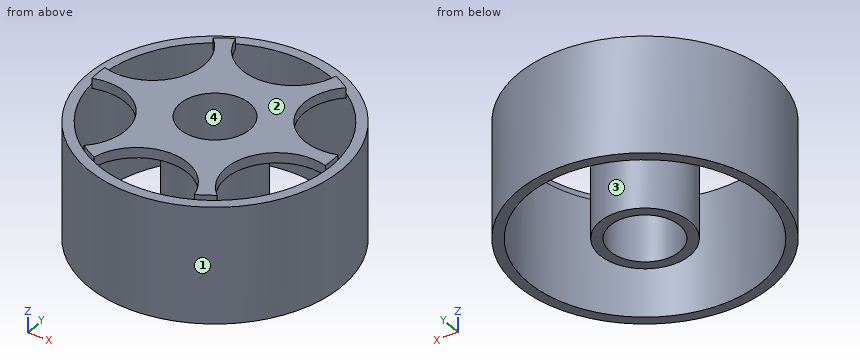
Autodesk Inventor part; units mm, degrees
ref_plane "YZ Plane" through (0, 0, 0) normal (1, 0, 0) x (0, 1, 0)
ref_plane "XZ Plane" through (0, 0, 0) normal (0, 1, 0) x (-1, 0, 0)
ref_plane "XY Plane" through (0, 0, 0) normal (0, 0, 1) x (1, 0, 0)
sketch "Sketch1" plane through (0, 0, 0) normal (0, 0, 1) x (1, 0, 0)
  circle A0 centre (0, 0) radius 5.588
  circle A1 centre (0, 0) radius 4.318
  circle A2 centre (0, 0) radius 14.478
  circle A3 centre (0, 0) radius 15.748
  dimension "d0" = 11.176
  dimension "d1" = 1.27
  dimension "d2" = 8.89
  dimension "d3" = 1.27
extrude "Extrusion1" add sketch "Sketch1" along normal blind 14.478
ref_plane "Work Plane1" through (0, 0, 14.478) normal (0, 0, 1) x (1, 0, 0)
sketch "Sketch2" plane through (0, 0, 14.478) normal (0, 0, 1) x (1, 0, 0)
  circle A0 centre (0, 0) radius 14.478
  circle A1 centre (0, 0) radius 15.748
  circle A2 centre (0, 0) radius 4.318
  circle A3 centre (0, 0) radius 5.588
extrude "Extrusion2" add sketch "Sketch2" along normal mid plane 1.27 contours A0 | A3
sketch "Sketch3" plane through (0, 0, 15.113) normal (0, 0, 1) x (1, 0, 0)
  circle A0 centre (0, 0) radius 14.478
  circle A1 centre (0, 0) radius 14.478
  arc A2 (-6.2546, 13.0573) -> (6.1362, 13.1134) centre (-0.0655, 14.4779) ccw
  arc A3 (6.1362, 13.1134) -> (-6.2546, 13.0573) centre (0, 0) ccw
  dimension "d9" = 12.7
extrude "Extrusion3" cut sketch "Sketch3" against normal blind 1.27 contours A2 A0 picked at (-1.876, 12.3773)
pattern_circular "Circular Pattern1" count 6 over 360 about axis through (0, 0, 14.478) along (0, 0, 1) of "Extrusion3"
properties part number "Wheel" material "ABS Plastic"
The listing builds one solid part. Answer for the finished solid, in the listing's coordinates (mm). Face numbers are marked on the shaded views. Round coordinates to 2 decimals unless told otherwise and drop trailing zeros. Loops run counter-clockwise (first coordinate to the right, second up) from the corner with the lowest first, then second, coordinate; pieces in that order, holes last. Notation, with made-up numbers: (20, -35.5) - (79, -35.5) arc R16 ccw to (79, -25.5) - close; hole circle Ø4 at (49, -15.75). An arc over 180 degrees is marked (long way). Return JSON: item names as keys, results as strings. Group by question number.
1. The part is cut by section D-D on y = -9.5. Determine the outline of the cut face in (x, z).
2. The mould has two halves that part along Y. Classify the marked faces 1, 2, 3 and 4: pulls with the +Y half, pulls with the -Y half, needs draft (parallel to the pull), parting line crosses it, or undercut.
3. Consider probe 1 along Y at (x, z) = (0, 6.75); probe 2 along X at (y, z) = (-11, 14); probe 3 along X at (y, z) = (1, 2.5). Determine where each line is inside the solid, lowest interval first.
4. The part is cut by section B-B on x = 0. Determine the outline of the cut face in (y, z).
5. Each of these flat-tipped pins is pushed along its axis until it touches: P1, Ø11, axis at x = 0, y = 0, coming from the -Z side; P2, Ø1, axis at y = 5.5, z = 13.5, coming from the +X side; P3, Ø2, axis at y = 3.5, z = 8, coming from the +X side; P4, Ø8, axis at x = -8.5, z = 3.5, coming from the +Y side. Where does it stop, or does it pass through?
6. The part is cut by section C-C on z = 9.75. Determine the outline of the cut face in (x, y), then the cut area to 3 significant figures.
7. The part is cut by section A-A on y = 0. Determine the outline of the cut face in (x, z).
Resolved:
{
 "1": {"outline": "(-12.56, 0) - (-10.93, 0) - (-10.93, 14.48) - (-12.56, 14.48) - close; (-6.55, 13.84) - (-3.88, 13.84) - (-3.88, 15.11) - (-6.55, 15.11) - close; (4.01, 13.84) - (6.66, 13.84) - (6.66, 15.11) - (4.01, 15.11) - close; (10.93, 0) - (12.56, 0) - (12.56, 14.48) - (10.93, 14.48) - close"},
 "2": {"face 1": "parting line crosses it", "face 2": "needs draft", "face 3": "undercut", "face 4": "undercut"},
 "3": {"probe 1": "y = -15.75 to -14.48, -5.59 to -4.32, 4.32 to 5.59, 14.48 to 15.75", "probe 2": "x = -11.27 to -9.41, -7.35 to -5.25, 5.38 to 7.5, 9.41 to 11.27", "probe 3": "x = -15.72 to -14.44, -5.5 to -4.2, 4.2 to 5.5, 14.44 to 15.72"},
 "4": {"outline": "(-15.75, 0) - (-14.48, 0) - (-14.48, 14.48) - (-15.75, 14.48) - close; (-8.13, 13.84) - (-5.59, 13.84) - (-5.59, 0) - (-4.32, 0) - (-4.32, 15.11) - (-8.13, 15.11) - close; (4.32, 0) - (5.59, 0) - (5.59, 13.84) - (8.13, 13.84) - (8.13, 15.11) - (4.32, 15.11) - close; (14.48, 0) - (15.75, 0) - (15.75, 14.48) - (14.48, 14.48) - close"},
 "5": {"P1": "stops at z = 0", "P2": "stops at x = 14.93", "P3": "stops at x = 15.55", "P4": "stops at y = 15.09"},
 "6": {"outline": "circle Ø31.5 at (0, 0); circle Ø11.18 at (0, 0); hole circle Ø28.96 at (0, 0); hole circle Ø8.64 at (0, 0)", "area": "160 mm²"},
 "7": {"outline": "(-15.75, 0) - (-14.48, 0) - (-14.48, 13.84) - (-5.59, 13.84) - (-5.59, 0) - (-4.32, 0) - (-4.32, 15.11) - (-14.48, 15.11) - (-14.48, 14.48) - (-15.75, 14.48) - close; (4.32, 0) - (5.59, 0) - (5.59, 13.84) - (14.48, 13.84) - (14.48, 0) - (15.75, 0) - (15.75, 14.48) - (14.48, 14.48) - (14.48, 15.11) - (4.32, 15.11) - close"}
}
